from build123d import *

# Parameters (mm, degrees)
BOSS_EXTRU_1_DEPTH = 3
CHANFREIN1_SIZE    = 5


with BuildPart() as part:
    # Esquisse1 → Boss.-Extru.1 (new body)
    with BuildSketch(Plane(origin=(0, 0, 0), x_dir=(1, 0, 0), z_dir=(0, 1, 0))):
        Polygon((0, 0), (-30.5, 0), (-30.5, 43), (-63.5, 43), (-63.5, 121), (63.5, 121), (63.5, 43), (30.5, 43), (30.5, 0), align=None)
    extrude(amount=BOSS_EXTRU_1_DEPTH)

    # Chanfrein1
    chanfrein1_edges = [part.edges().sort_by_distance(p)[0] for p in [
        (-63.5, 1.5, -43),
        (-63.5, 1.5, -121),
        (63.5, 1.5, -121),
        (63.5, 1.5, -43),
    ]]
    chamfer(chanfrein1_edges, length=CHANFREIN1_SIZE)


solid = part.part
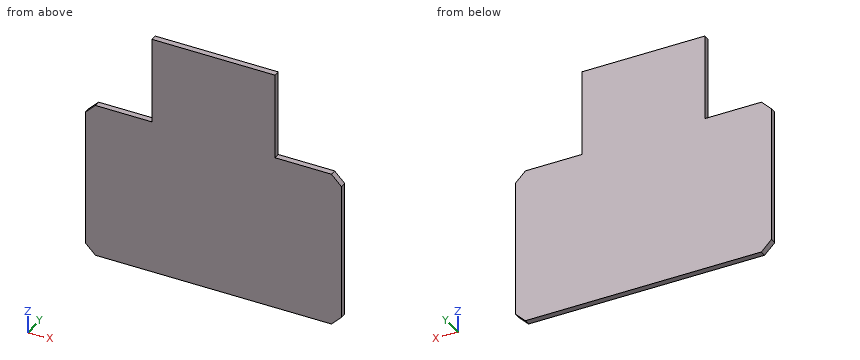
Here's how the part is built. I have some questions about the finished solid (model axes, mm). Give positions to 0.01 mm unless a question says otherwise; leave off trailing zeros. Write each loop counter-clockwise with the first axis right and the second up, starting at its lowest first coordinate (ties: lowest second). Pieces come first, ordered by that corner, then holes. Notation, with made-up numbers: (-29, -11.75) -> (9, -11.75) arc R24 ccw to (9, 17.25) -> close; hole circle Ø5 at (-2, -3). An arc over 180 degrees is marked (long way). Use one line per item in the form item = value. Start each with the question number.
1. If I drill on L1, parallel to Z at x = -50, y = 0.85; L2, parallel to X at y = 1.45, z = -39, over which ranges is the centre line in solid material (lowest first)?
2. Will these pins go through, and if not, where does the flat tip stop? pin 1 Ø1.5 at (x, y) = (45.5, 1.5) entering from +Z; pin 2 Ø0.9 at (y, z) = (2, -16) entering from -X; pin 3 Ø1.5 at (y, z) = (1.5, -21) entering from +X.
3. Imagine slicing it at A-A on y = 2. List the corners of the cut face in (x, z) for me, plus the area to 3 significant figures.
4. Imagine slicing it at B-B on x = -53. List the corners of the cut face in (y, z) for me.
Entries:
q1.L1 = -121 to -43
q1.L2 = -30.5 to 30.5
q2.pin_1 = -43
q2.pin_2 = -30.5
q2.pin_3 = 30.5
q3.outline = (-63.5, -116) -> (-58.5, -121) -> (58.5, -121) -> (63.5, -116) -> (63.5, -48) -> (58.5, -43) -> (30.5, -43) -> (30.5, 0) -> (-30.5, 0) -> (-30.5, -43) -> (-58.5, -43) -> (-63.5, -48) -> close
q3.area = 12,500 mm²
q4.outline = (0, -121) -> (3, -121) -> (3, -43) -> (0, -43) -> close
